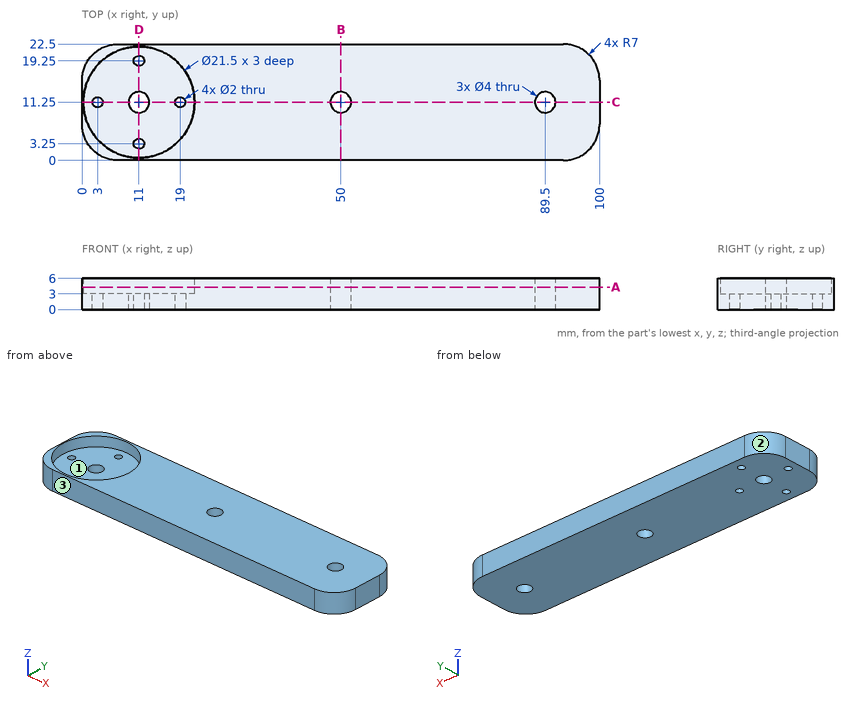
Could you check a few things on this drawing? It's one solid part, dimensions in mm from its lowest x, y, z. Round coordinates to 2 decimals unless told otherwise and drop trailing zeros. Write each loop counter-clockwise with the first axis right and the second up, starting at its lowest first coordinate (ties: lowest second). Pieces come first, ordered by that corner, then holes. Notation, with made-up numbers: M 45.5,33.25 L 75.5,33.25 A24 ccw 75.5,50.25 Z; hole C 7,71.25 d10. An arc over 180 degrees is marked long. Answer as CSV lines item,"result". Start each with the question number.
1. I need wall thicknesses on probe 1 along Y at (x, z) = (11, 1.1); probe 2 along X at (y, z) = (12.25, 4.6); probe 3 along Y at (x, z) = (19, 0.6). Which ranges of each line are inside material? Lowest first, please.
2. I'm going to push flat-ended pins straight in: pin 1 Ø3 at (x, y) = (11, 3.25) entering from +Z; pin 2 Ø3 at (y, z) = (20, 5) entering from +X. Where does each tip first touch, or does it pass through?
3. Suppose I cut it at C-C on y = 11.25. Write out the boundary of the cut face in (x, z).
4. Suppose I cut it at A-A on z = 4.3. Write out the boundary of the cut face in (x, y).
5. Thinking about a two-plate mould opening in X: for the marked faces 1, 2 and 3, which applies, released by +X, released by -X, zero draft, split by the parting line, or undercut?
6. Suppose I cut it at D-D on x = 11. Write out the boundary of the cut face in (y, z), then the cut area to 3 significant figures.
7. Suppose I cut it at B-B on x = 50. Write out the boundary of the cut face in (y, z), then the cut area to 3 significant figures.
Check result:
1,probe 1,"y = 0 to 2.25, 4.25 to 9.25, 13.25 to 18.25, 20.25 to 22.5"
1,probe 2,"x = 0 to 0.3, 21.7 to 48.27, 51.73 to 87.77, 91.23 to 100"
1,probe 3,"y = 0 to 10.25, 12.25 to 22.5"
2,pin 1,"stops at z = 3"
2,pin 2,"stops at x = 99.32"
3,outline,"M 0,0 L 2,0 L 2,3 L 0.25,3 L 0.25,6 L 0,6 Z; M 4,0 L 9,0 L 9,3 L 4,3 Z; M 13,0 L 18,0 L 18,3 L 13,3 Z; M 20,0 L 48,0 L 48,6 L 21.75,6 L 21.75,3 L 20,3 Z; M 52,0 L 87.5,0 L 87.5,6 L 52,6 Z; M 91.5,0 L 100,0 L 100,6 L 91.5,6 Z"
4,outline,"M 0,7 A7 ccw 7,0 L 93,0 A7 ccw 100,7 L 100,15.5 A7 ccw 93,22.5 L 7,22.5 A7 ccw 0,15.5 Z; hole C 11,11.25 d21.5; hole C 50,11.25 d4; hole C 89.5,11.25 d4"
5,face 1,"undercut"
5,face 2,"released by -X"
5,face 3,"zero draft"
6,outline,"M 0,0 L 2.25,0 L 2.25,3 L 0.5,3 L 0.5,6 L 0,6 Z; M 4.25,0 L 9.25,0 L 9.25,3 L 4.25,3 Z; M 13.25,0 L 18.25,0 L 18.25,3 L 13.25,3 Z; M 20.25,0 L 22.5,0 L 22.5,6 L 22,6 L 22,3 L 20.25,3 Z"
6,area,"46.5 mm2"
7,outline,"M 0,0 L 9.25,0 L 9.25,6 L 0,6 Z; M 13.25,0 L 22.5,0 L 22.5,6 L 13.25,6 Z"
7,area,"111 mm2"
